Autodesk Inventor part; units mm, degrees
ref_plane "YZ Plane" through (0, 0, 0) normal (1, 0, 0) x (0, 1, 0)
ref_plane "XZ Plane" through (0, 0, 0) normal (0, 1, 0) x (-1, 0, 0)
ref_plane "XY Plane" through (0, 0, 0) normal (0, 0, 1) x (1, 0, 0)
ref_plane "Płaszczyzna konstrukcyjna1" through (0, 19, 0) normal (0, 1, 0) x (1, 0, 0)
sketch "Szkic21" plane through (0, 19, 0) normal (0, 1, 0) x (1, 0, 0)
  line L0 (-5.3, -65.6) -> (-5.3, -67.6)
  line L1 (-25.3, -67.6) -> (-5.3, -67.6)
  line L2 (0, -65.6) -> (-5.3, -65.6)
  line L3 (-5.3, -67.6) -> (-5.3, -65.6)
  line L4 (-5.3, -65.6) -> (0, -65.6)
  line L5 (0, 0) -> (0, -65.6)
  line L6 (0, -65.6) -> (0, 0)
  line L7 (-30.6, -65.6) -> (-30.6, 0)
  line L8 (0, 0) -> (-30.6, 0)
  line L9 (-30.6, 0) -> (-30.6, -65.6)
  line L10 (-25.3, -67.6) -> (-25.3, -65.6)
  line L11 (-30.6, -65.6) -> (-25.3, -65.6)
  line L12 (-25.3, -65.6) -> (-25.3, -67.6)
  line L13 (-30.6, -65.6) -> (-29.1, -65.6) construction
  line L14 (-29.1, -65.6) -> (-29.1, -64.1) construction
  line L15 (-29.1, -64.1) -> (-30.6, -64.1) construction
  line L16 (-30.6, -64.1) -> (-30.6, -65.6) construction
  line L17 (-30.6, 0) -> (-29.1, 0) construction
  line L18 (-29.1, 0) -> (-29.1, -1.5) construction
  line L19 (-29.1, -1.5) -> (-30.6, -1.5) construction
  line L20 (-30.6, -1.5) -> (-30.6, 0) construction
  line L21 (0, 0) -> (-1.5, 0) construction
  line L22 (-1.5, 0) -> (-1.5, -1.5) construction
  line L23 (-1.5, -1.5) -> (0, -1.5) construction
  line L24 (0, -1.5) -> (0, 0) construction
  line L25 (0, -65.6) -> (-1.5, -65.6) construction
  line L26 (-1.5, -65.6) -> (-1.5, -64.1) construction
  line L27 (-1.5, -64.1) -> (0, -64.1) construction
  line L28 (0, -64.1) -> (0, -65.6) construction
  line L29 (-5.3, -65.6) -> (-6.8, -65.6) construction
  line L30 (-6.8, -65.6) -> (-6.8, -64.1) construction
  line L31 (-6.8, -64.1) -> (-5.3, -64.1) construction
  line L32 (-5.3, -64.1) -> (-5.3, -65.6) construction
  line L33 (-5.3, -67.6) -> (-6.8, -67.6) construction
  line L34 (-6.8, -67.6) -> (-6.8, -66.1) construction
  line L35 (-6.8, -66.1) -> (-5.3, -66.1) construction
  line L36 (-5.3, -66.1) -> (-5.3, -67.6) construction
  line L37 (-21.8, -67.6) -> (-25.3, -67.6) construction
  line L38 (-25.3, -67.6) -> (-23.8, -67.6) construction
  line L39 (-23.8, -67.6) -> (-23.8, -66.1) construction
  line L40 (-23.8, -66.1) -> (-25.3, -66.1) construction
  line L41 (-25.3, -66.1) -> (-25.3, -67.6) construction
  line L42 (-25.3, -65.6) -> (-23.8, -65.6) construction
  line L43 (-23.8, -65.6) -> (-23.8, -64.1) construction
  line L44 (-23.8, -64.1) -> (-25.3, -64.1) construction
  line L45 (-25.3, -64.1) -> (-25.3, -65.6) construction
  line L46 (-29.1, -64.1) -> (-29.1, -1.5)
  line L47 (-29.1, -1.5) -> (-1.5, -1.5)
  line L48 (-1.5, -1.5) -> (-1.5, -64.1)
  line L49 (-1.5, -64.1) -> (-6.8, -64.1)
  line L50 (-6.8, -64.1) -> (-6.8, -66.1)
  line L51 (-6.8, -66.1) -> (-23.8, -66.1)
  line L52 (-23.8, -66.1) -> (-23.8, -64.1)
  line L53 (-23.8, -64.1) -> (-29.1, -64.1)
  dimension "d115" = 1.5
  dimension "d116" = 1.5
  dimension "d117" = 1.5
  dimension "d118" = 1.5
  dimension "d119" = 1.5
  dimension "d120" = 1.5
  dimension "d121" = 1.5
  dimension "d122" = 1.5
  dimension "d123" = 1.5
  dimension "d124" = 1.5
  dimension "d125" = 1.5
  dimension "d126" = 1.5
  dimension "d127" = 1.5
  dimension "d128" = 1.5
  dimension "d129" = 1.5
  dimension "d130" = 1.5
extrude "Wyciągnięcie proste19" add sketch "Szkic21" against normal blind 2
ref_plane "Płaszczyzna konstrukcyjna3" through (0, 19, 0) normal (0, 1, 0) x (1, 0, 0)
sketch "Szkic22" plane through (0, 19, 0) normal (0, 1, 0) x (1, 0, 0)
  line L0 (1.5, -67.6) -> (1.5, 1.5)
  line L1 (1.5, -67.6) -> (1.5, 1.5)
  line L2 (1.5, 1.5) -> (-32.1, 1.5)
  line L3 (1.5, 1.5) -> (-32.1, 1.5)
  line L4 (-32.1, -67.6) -> (-26.8, -67.6)
  line L5 (-32.1, 1.5) -> (-32.1, -67.6)
  line L6 (-32.1, -67.6) -> (-26.8, -67.6)
  line L7 (-26.8, -69.1) -> (-23.3, -69.1)
  line L8 (-26.8, -67.6) -> (-26.8, -69.1)
  line L9 (-7.3, -69.1) -> (-3.8, -69.1)
  line L10 (-26.8, -69.1) -> (-3.8, -69.1)
  line L11 (-3.8, -69.1) -> (-3.8, -67.6)
  line L12 (-3.8, -67.6) -> (1.5, -67.6)
  line L13 (-3.8, -67.6) -> (1.5, -67.6)
  point P0 (0, 0)
extrude "Wyciągnięcie proste20" add sketch "Szkic22" along normal blind 1.5
ref_plane "Płaszczyzna konstrukcyjna2" through (0, 24, 0) normal (0, 1, 0) x (1, 0, 0)
ref_plane "Płaszczyzna konstrukcyjna5" through (0, 24, 0) normal (0, 1, 0) x (1, 0, 0)
ref_plane "Płaszczyzna konstrukcyjna6" through (0, 24, 0) normal (0, 1, 0) x (1, 0, 0)
ref_plane "Płaszczyzna konstrukcyjna4" through (0, 20.5, 0) normal (0, 1, 0) x (1, 0, 0)
sketch "Szkic26" plane through (0, 20.5, 0) normal (0, 1, 0) x (1, 0, 0)
  line L0 (1.5, -67.6) -> (1.5, 1.5) construction
  line L1 (1.5, 1.5) -> (1.5, -0.3) construction
  line L2 (1.5, -0.3) -> (1.5, -25.3) construction
  line L3 (1.5, -0.3) -> (1.5, -48.3) construction
  line L4 (1.5, -48.3) -> (0, -48.3) construction
  line L5 (0, -48.3) -> (-7, -48.3)
  line L6 (-7, -48.3) -> (-7, -25.3)
  line L7 (-7, -25.3) -> (0, -25.3)
  line L8 (0, -25.3) -> (0, -48.3)
  point P0 (0, 0)
  dimension "d146" = 1.8
  dimension "d147" = 25
  dimension "d148" = 48
  dimension "d149" = 7
extrude "Wyciągnięcie proste24" cut sketch "Szkic26" against normal blind 5
sketch "Szkic28" plane through (0, 20.5, 0) normal (0, 1, 0) x (1, 0, 0)
  line L0 (-32.1, -67.6) -> (-26.8, -67.6) construction
  line L1 (-32.1, -67.6) -> (-24.1, -67.6) construction
  line L2 (-24.1, -67.6) -> (-22.1, -67.6) construction
  line L3 (-23.3, -67.6) -> (-7.3, -67.6) construction
  line L4 (-24.1, -67.6) -> (-24.1, -69.1) construction
  line L5 (-26.8, -69.1) -> (-3.8, -69.1) construction
  line L6 (-24.1, -69.1) -> (-24.1, -62.1) construction
  line L7 (-24.1, -62.1) -> (-24.1, -58.1) construction
  line L8 (-24.1, -62.1) -> (-22.1, -62.1) construction
  line L9 (-22.1, -62.1) -> (-24.1, -62.1)
  line L10 (-24.1, -62.1) -> (-24.1, -58.1)
  line L11 (-24.1, -58.1) -> (-22.1, -58.1)
  line L12 (-22.1, -58.1) -> (-22.1, -62.1)
  point P0 (0, 0)
  dimension "d158" = 8
  dimension "d159" = 2
  dimension "d160" = 7
  dimension "d161" = 4
  dimension "d162" = 2
extrude "Wyciągnięcie proste26" cut sketch "Szkic28" against normal blind 10
properties part number "goraczesc2zotworem"
Build history of the part. All positions in model axes, mm. A direction names the side the tool comes from. Round coordinates to 2 decimals unless told otherwise and drop trailing zeros. Order: outer loops, then holes, each group sorted by start corner. A loop starts at its lowest first (then second) coordinate and runs counter-clockwise, first axis right, second up. Notation, with made-up numbers: M 41,89.25 L 99,89.25 A12 ccw 99,102.25 Z; hole C 48,-33.75 d4. An arc over 180 degrees is marked long. Use CSV: the item, a comma, the result in double quotes. Start each with the question number.
(1) Tool access for faces 4 (the face through (-5.3, 18, 67)), 5 (the face through (-26.8, 20, 68)), 6 (the face through (-22.1, 20, 60)), 7 (the face through (-6.8, 18, 65)): list every direction of +Z, -Z, +X, -X, +Y, -Y with a clear straight run to the whole face (end or side of a thin tool).
(2) Cut at C-C on x = -10. List the corners of the cut face in (y, z).
(3) Cut at D-D on z = 49. List the corners of the cut face in (x, y), then the cut area to 3 significant figures.
(4) Flat gauge pins, fed straight in: P1, Ø0.6, axis at y = 18, z = 67, coming from the -X side; P2, Ø1.6, axis at y = 17.5, z = 65, coming from the -X side; P3, Ø0.6, axis at x = -16, y = 17.5, coming from the -Z side. Where does each tip first touch, or does it go through?
(5) Drill centre lines: probe 1 along Z at (x, y) = (-12.5, 17.85); probe 2 along X at (y, z) = (18.65, 14); probe 3 along Z at (x, y) = (-4, 18.65). Where is each one in solid material? Low to high.
(6) Cut at B-B on y = 19.7. List the corners of the cut face in (x, z), then the cut area to 3 significant figures.
(7) Mould opens along Z. For faces 1 (the face through (-24.1, 20, 60)), 2 (the face through (-15, 18, 67.6)), 3 (the face through (-32.1, 20, 33)) say: +Z half, -Z half, draft (parallel to the pull), parting line (faces both ways), or undercut.
(8) Cut at A-A on z = 35. List the corners of the cut face in (x, y).
Findings:
1,face 4,"+Z, +X, -Y"
1,face 5,"+Z, -X, +Y, -Y"
1,face 6,"+Y, -Y"
1,face 7,"-Y"
2,outline,"M 17,0 L 19,0 L 19,-1.5 L 20.5,-1.5 L 20.5,69.1 L 19,69.1 L 19,67.6 L 17,67.6 L 17,66.1 L 19,66.1 L 19,1.5 L 17,1.5 Z"
3,outline,"M -32.1,19 L -30.6,19 L -30.6,17 L -29.1,17 L -29.1,19 L -1.5,19 L -1.5,17 L 0,17 L 0,19 L 1.5,19 L 1.5,20.5 L -32.1,20.5 Z"
3,area,"56.4 mm^2"
4,P1,"stops at x = -25.3"
4,P2,"stops at x = -30.6"
4,P3,"stops at z = 0"
5,probe 1,"z = 0 to 1.5, 66.1 to 67.6"
5,probe 2,"x = -30.6 to -29.1, -1.5 to 0"
5,probe 3,"z = 0 to 1.5, 64.1 to 65.6"
6,outline,"M -32.1,-1.5 L 1.5,-1.5 L 1.5,67.6 L -3.8,67.6 L -3.8,69.1 L -26.8,69.1 L -26.8,67.6 L -32.1,67.6 Z; hole M -24.1,58.1 L -22.1,58.1 L -22.1,62.1 L -24.1,62.1 Z; hole M -7,25.3 L 0,25.3 L 0,48.3 L -7,48.3 Z"
6,area,"2,190 mm^2"
7,face 1,"undercut"
7,face 2,"+Z half"
7,face 3,"draft"
8,outline,"M -32.1,19 L -30.6,19 L -30.6,17 L -29.1,17 L -29.1,19 L -7,19 L -7,20.5 L -32.1,20.5 Z; M 0,19 L 1.5,19 L 1.5,20.5 L 0,20.5 Z"
